```python
from build123d import *

# Parameters (mm, degrees)
EXTRUDE_1_DEPTH     = 4
CUT_EXTRUDE_1_DEPTH = 1
SKETCH_3_R          = 3.75
SKETCH_3_R_2        = 1.75
EXTRUDE_2_DEPTH     = 1
FILLET_1_R          = 1


with BuildPart() as part:
    # 草图1 → 凸台-拉伸1 (new body)
    with BuildSketch(Plane(origin=(0, 0, 0), x_dir=(1, 0, 0), z_dir=(0, 1, 0))):
        Polygon((14.43375673, 0), (7.216878365, 12.5), (-7.216878365, 12.5), (-14.43375673, 0), (-7.216878365, -12.5), (7.216878365, -12.5), align=None)
    extrude(amount=EXTRUDE_1_DEPTH)

    # 草图2 → 切除-拉伸1 (cut)
    with BuildSketch(Plane(origin=(0, 4, 0), x_dir=(1, 0, 0), z_dir=(0, 1, 0))):
        Polygon((5.484827557, -9.5), (10.969655115, 0), (5.484827557, 9.5), (-5.484827557, 9.5), (-10.969655115, 0), (-5.484827557, -9.5), align=None)
    extrude(amount=-CUT_EXTRUDE_1_DEPTH, mode=Mode.SUBTRACT)

    # 草图3 → 凸台-拉伸2 (add)
    # profile 1 of 2: a face of its own
    with BuildSketch(Plane(origin=(0, 3, 0), x_dir=(1, 0, 0), z_dir=(0, 1, 0))):
        with BuildLine():
            Line((8.124640736, -0.490115197), (7.750329512, 2.486441724))
            Line((7.750329512, 2.486441724), (5.47592438, 2.452397232))
            ThreePointArc((5.47592438, 2.452397232), (5.213474627, 2.969794996), (4.902281736, 3.4594268))
            Line((4.902281736, 3.4594268), (6.091552339, 5.39842478))
            Line((6.091552339, 5.39842478), (3.72213075, 7.238490359))
            Line((3.72213075, 7.238490359), (2.137956549, 5.606169975))
            ThreePointArc((2.137956549, 5.606169975), (1.586521082, 5.786445442), (1.02025251, 5.912620808))
            Line((1.02025251, 5.912620808), (0.490115197, 8.124640736))
            Line((0.490115197, 8.124640736), (-2.486441724, 7.750329512))
            Line((-2.486441724, 7.750329512), (-2.452397232, 5.47592438))
            ThreePointArc((-2.452397232, 5.47592438), (-2.969794996, 5.213474627), (-3.4594268, 4.902281736))
            Line((-3.4594268, 4.902281736), (-5.39842478, 6.091552339))
            Line((-5.39842478, 6.091552339), (-7.238490359, 3.72213075))
            Line((-7.238490359, 3.72213075), (-5.606169975, 2.137956549))
            ThreePointArc((-5.606169975, 2.137956549), (-5.786445442, 1.586521082), (-5.912620808, 1.02025251))
            Line((-5.912620808, 1.02025251), (-8.124640736, 0.490115197))
            Line((-8.124640736, 0.490115197), (-7.750329512, -2.486441724))
            Line((-7.750329512, -2.486441724), (-5.47592438, -2.452397232))
            ThreePointArc((-5.47592438, -2.452397232), (-5.213474627, -2.969794996), (-4.902281736, -3.4594268))
            Line((-4.902281736, -3.4594268), (-6.091552339, -5.39842478))
            Line((-6.091552339, -5.39842478), (-3.72213075, -7.238490359))
            Line((-3.72213075, -7.238490359), (-2.137956549, -5.606169975))
            ThreePointArc((-2.137956549, -5.606169975), (-1.586521082, -5.786445442), (-1.02025251, -5.912620808))
            Line((-1.02025251, -5.912620808), (-0.490115197, -8.124640736))
            Line((-0.490115197, -8.124640736), (2.486441724, -7.750329512))
            Line((2.486441724, -7.750329512), (2.452397232, -5.47592438))
            ThreePointArc((2.452397232, -5.47592438), (2.969794996, -5.213474627), (3.4594268, -4.902281736))
            Line((3.4594268, -4.902281736), (5.39842478, -6.091552339))
            Line((5.39842478, -6.091552339), (7.238490359, -3.72213075))
            Line((7.238490359, -3.72213075), (5.606169975, -2.137956549))
            ThreePointArc((5.606169975, -2.137956549), (5.786445442, -1.586521082), (5.912620808, -1.02025251))
            Line((5.912620808, -1.02025251), (8.124640736, -0.490115197))
        make_face()
        with Locations(Location((0, 0, 0), (0, 0, 270))):
            Circle(SKETCH_3_R, mode=Mode.SUBTRACT)
    # profile 2 of 2: a face of its own
    with BuildSketch(Plane(origin=(0, 3, 0), x_dir=(1, 0, 0), z_dir=(0, 1, 0))):
        with Locations(Location((0, 0, 0), (0, 0, 270))):
            Circle(SKETCH_3_R_2)
    extrude(amount=EXTRUDE_2_DEPTH)

    # 圆角1
    fillet_1_edges = [part.edges().sort_by_distance(p)[0] for p in [
        (7.216878365, 2, 12.5),
        (-7.216878365, 2, 12.5),
        (-14.43375673, 2, 0),
        (-7.216878365, 2, -12.5),
        (7.216878365, 2, -12.5),
        (14.43375673, 2, 0),
        (5.484827557, 3.5, 9.5),
        (-5.484827557, 3.5, 9.5),
        (-10.969655115, 3.5, 0),
        (-5.484827557, 3.5, -9.5),
        (5.484827557, 3.5, -9.5),
        (10.969655115, 3.5, 0),
    ]]
    fillet(fillet_1_edges, radius=FILLET_1_R)


solid = part.part
```
Build history of the part. All positions in model axes, mm. A direction names the side the tool comes from. Give positions to 0.01 mm unless a question says otherwise; leave off trailing zeros. Loops run counter-clockwise (first coordinate to the right, second up) from the corner with the lowest first, then second, coordinate; pieces in that order, holes last. Notation, with made-up numbers: (-12, -37.75) - (44, -37.75) arc R31 cw to (44, -0.75) - close; hole circle Ø11 at (19.25, 56.5). An arc over 180 degrees is marked (long way). Use a Markdown table: item, result.
(1) Wall check: line 1 along X through (y, z) = (3.15, 3); line 2 along X through (y, z) = (3.4, 0); line 3 along Y through (x, z) = (-7.75, -2.25). Give the ranges that are in metal, low to high.
Taken from the geometry:
| item | result |
|---|---|
| line 1 | -12.7 to -9.24, -5.2 to -2.25, 2.25 to 6.49, 9.24 to 12.7 |
| line 2 | -14.28 to -10.81, -8.06 to -3.75, -1.75 to 1.75, 3.75 to 8.06, 10.81 to 14.28 |
| line 3 | 0 to 3 |
(2) Band-saw the part on B-B (z = 0). Give the cut face in (x, y).
Taken from the geometry:
| item | result |
|---|---|
| outline | (-14.28, 0) - (14.28, 0) - (14.28, 4) - (10.81, 4) - (10.81, 3) - (8.06, 3) - (8.06, 4) - (3.75, 4) - (3.75, 3) - (1.75, 3) - (1.75, 4) - (-1.75, 4) - (-1.75, 3) - (-3.75, 3) - (-3.75, 4) - (-8.06, 4) - (-8.06, 3) - (-10.81, 3) - (-10.81, 4) - (-14.28, 4) - close |
(3) Drop flat-ended pins along their axis: pin 1 Ø1.5 at (y, z) = (1.5, -2) entering from +X; pin 2 Ø2 at (x, y) = (7.5, 0.5) entering from +Z; pin 3 Ø2 at (x, y) = (8, 2.5) entering from +Z. Give the stop position or say it passes through.
Taken from the geometry:
| item | result |
|---|---|
| pin 1 | x = 13.71 |
| pin 2 | z = 12.5 |
| pin 3 | z = 12.43 |
(4) Band-saw the part on A-A (y = 1.5). Give the cut face in (x, z).
Taken from the geometry:
| item | result |
|---|---|
| outline | (-14.15, -0.5) - (-7.51, -12) arc R1 ccw to (-6.64, -12.5) - (6.64, -12.5) arc R1 ccw to (7.51, -12) - (14.15, -0.5) arc R1 ccw to (14.15, 0.5) - (7.51, 12) arc R1 ccw to (6.64, 12.5) - (-6.64, 12.5) arc R1 ccw to (-7.51, 12) - (-14.15, 0.5) arc R1 ccw to start |
(5) Band-saw the part on C-C (x = 0). Give the cut face in (y, z), and give its area (3 significant figures).
Taken from the geometry:
| item | result |
|---|---|
| outline | (0, -12.5) - (4, -12.5) - (4, -9.5) - (3, -9.5) - (3, -8.06) - (4, -8.06) - (4, -3.75) - (3, -3.75) - (3, -1.75) - (4, -1.75) - (4, 1.75) - (3, 1.75) - (3, 3.75) - (4, 3.75) - (4, 8.06) - (3, 8.06) - (3, 9.5) - (4, 9.5) - (4, 12.5) - (0, 12.5) - close |
| area | 93.1 mm2 |
(6) Which spindle directions (+Z, -Z, +X, -X, +Y, -Y) get a long thin tool onto all of the face, cutting with end or side? Do faces 4 (the face through (-1.594, 3.493, 5.784)), 5 (the face through (10.78, 1.97, 6.33)). Say none if no direction does.
Taken from the geometry:
| item | result |
|---|---|
| face 4 | +Y |
| face 5 | +Z, +X, +Y, -Y |
(7) Pull direction Z, two halves, no side cores. Call faces 1 (the face through (-7.13, 2.03, 12.37)), 2 (the face through (10.87, 1.97, -6.17)), 3 (the face through (-5.414, 3.493, 9.362)): +Z half, -Z half, draft (parallel to the pull), parting line (faces both ways), or undercut.
Taken from the geometry:
| item | result |
|---|---|
| face 1 | +Z half |
| face 2 | -Z half |
| face 3 | undercut |
